Autodesk Inventor part; units mm, degrees
ref_plane "YZ Plane" through (0, 0, 0) normal (1, 0, 0) x (0, 1, 0)
ref_plane "XZ Plane" through (0, 0, 0) normal (0, 1, 0) x (-1, 0, 0)
ref_plane "XY Plane" through (0, 0, 0) normal (0, 0, 1) x (1, 0, 0)
sketch "Sketch1" plane through (0, 0, 0) normal (0, 1, 0) x (-1, 0, 0)
  line L0 (-9.525, 9.525) -> (9.525, 9.525)
  line L1 (9.525, 9.525) -> (9.525, -9.525)
  line L2 (9.525, -9.525) -> (-9.525, -9.525)
  line L3 (-9.525, -9.525) -> (-9.525, 9.525)
  point P0 (0, 0)
  dimension "d0" = 19.05
  dimension "d1" = 19.05
  dimension "d2" = 9.525
  dimension "d3" = 9.525
extrude "Extrusion1" add sketch "Sketch1" along normal blind 6.35
sketch "Sketch2" plane through (0, 6.35, 0) normal (0, 1, 0) x (1, 0, 0)
  line L0 (-3.175, 1.905) -> (3.175, 1.905)
  line L1 (3.175, 1.905) -> (3.175, 0.762)
  line L2 (3.175, 0.762) -> (-3.175, 0.762)
  line L3 (-3.175, 0.762) -> (-3.175, 1.905)
  line L4 (-3.175, -0.762) -> (3.175, -0.762)
  line L5 (3.175, -0.762) -> (3.175, -1.905)
  line L6 (3.175, -1.905) -> (-3.175, -1.905)
  line L7 (-3.175, -1.905) -> (-3.175, -0.762)
  line L8 (0, 1.905) -> (0, 0.762)
  line L9 (0, -1.905) -> (0, -0.762)
  point P0 (0, 0)
  dimension "d6" = 6.35
  dimension "d7" = 1.143
  dimension "d8" = 3.175
  dimension "d11" = 1.524
  dimension "d12" = 0.762
  dimension "d13" = 6.35
  dimension "d14" = 1.143
extrude "Extrusion2" cut sketch "Sketch2" against normal blind 1.143 contours L0 L8 L2 L3 | L4 L9 L6 L7
extrude "Extrusion3" cut sketch "Sketch2" against normal blind 2.286 contours L0 L1 L2 L8 | L4 L5 L6 L9
sketch "Sketch3" plane through (0, 6.35, 0) normal (0, 1, 0) x (1, 0, 0)
  line L0 (0, -0.762) -> (0, -1.905)
  circle A0 centre (0, -1.3335) radius 0.5715
  line L1 (0, 0.762) -> (0, 1.905)
  circle A1 centre (0, 1.3335) radius 0.5715
  point P0 (0, 0)
extrude "Extrusion4" cut sketch "Sketch3" against normal through all
fillet "Fillet1" radius 3.175 4 edges at (-9.525, 3.175, 9.525) (9.525, 3.175, 9.525) (9.525, 3.175, -9.525) (-9.525, 3.175, -9.525)
properties part number "Unit_v2"
Input: part model. Units: mm. Frame: model coordinates. A direction names the side the tool comes from. Coordinates: 2 decimals unless noted, no trailing zeros. Write each loop counter-clockwise with the first axis right and the second up, starting at its lowest first coordinate (ties: lowest second). Pieces come first, ordered by that corner, then holes.
1) Section B-B on y = 5.5. Output: boundary loops of the cut face in (x, z) (3 decimals), and give its area (3 significant figures).
2) Section C-C on x = 2.25. Output: boundary loops of the cut face in (y, z) (3 decimals).
3) Set-up query: faces 5 (the flat face through (-2, 5.207, 1)), 6 (the flat face through (0, 3, 9.525)). Return all of +Z, -Z, +X, -X, +Y, -Y with unobstructed straight access to the full face (end or side cutting, diameter ignored); none if empty.
4) Section A-A on x = 0.25. Output: boundary loops of the cut face in (y, z) (3 decimals).
5) Pin query (flat end, axial travel): pin 1 Ø0.9 at (x, z) = (-2.5, 1) entering from +Y; pin 2 Ø1 at (x, y) = (-7, 1) entering from +Z. Return the tip coordinate at first contact, or that it passes through.
6) Section D-D on y = 2. State how many separate pieces and enclosed holes the cut face has, and give its area (3 significant figures).
7) Mould query, pull axis Z, two halves, no side actions, for faces 1 (the flat face through (0, 0, 0)), 2 (the flat face through (1, 5, -1.905)), 3 (the flat face through (1, 5, -0.762)), 4 (the cylindrical face through (8.62, 3.22, -8.57)). Classes: pulls with the +Z half, pulls with the -Z half, needs draft (parallel to the pull), parting line crosses it, or undercut.
8) Material intervals for line 1 along Z through (x, y) = (1, 5) (3 decimals); line 2 along X through (y, z) = (1, 1.25) (3 decimals); line 3 along Y through (x, z) = (2.5, -1.5), sorted ascending.
Check result:
1. outline: (-9.525, -6.35) arc R3.175 ccw to (-6.35, -9.525) - (6.35, -9.525) arc R3.175 ccw to (9.525, -6.35) - (9.525, 6.35) arc R3.175 ccw to (6.35, 9.525) - (-6.35, 9.525) arc R3.175 ccw to (-9.525, 6.35) - close; hole (-3.175, -1.905) - (3.175, -1.905) - (3.175, -0.762) - (-3.175, -0.762) - close; hole (-3.175, 0.762) - (3.175, 0.762) - (3.175, 1.905) - (-3.175, 1.905) - close
1. area: 340 mm2
2. outline: (0, -9.525) - (6.35, -9.525) - (6.35, -1.905) - (4.064, -1.905) - (4.064, -0.762) - (6.35, -0.762) - (6.35, 0.762) - (4.064, 0.762) - (4.064, 1.905) - (6.35, 1.905) - (6.35, 9.525) - (0, 9.525) - close
3. face 5: +Y
3. face 6: +Z, +X, -X, +Y, -Y
4. outline: (0, -9.525) - (6.35, -9.525) - (6.35, -1.905) - (4.064, -1.905) - (4.064, -1.847) - (0, -1.847) - close; (0, -0.82) - (4.064, -0.82) - (4.064, -0.762) - (6.35, -0.762) - (6.35, 0.762) - (4.064, 0.762) - (4.064, 0.82) - (0, 0.82) - close; (0, 1.847) - (4.064, 1.847) - (4.064, 1.905) - (6.35, 1.905) - (6.35, 9.525) - (0, 9.525) - close
5. pin 1: stops at y = 6.35
5. pin 2: stops at z = 9.52
6. separate pieces: 1
6. enclosed holes: 2
6. area: 352 mm2
7. face 1: needs draft
7. face 2: undercut
7. face 3: undercut
7. face 4: pulls with the -Z half
8. line 1: z = -9.525 to -1.905, -0.762 to 0.762, 1.905 to 9.525
8. line 2: x = -9.525 to -0.565, 0.565 to 9.525
8. line 3: y = 0 to 4.06
